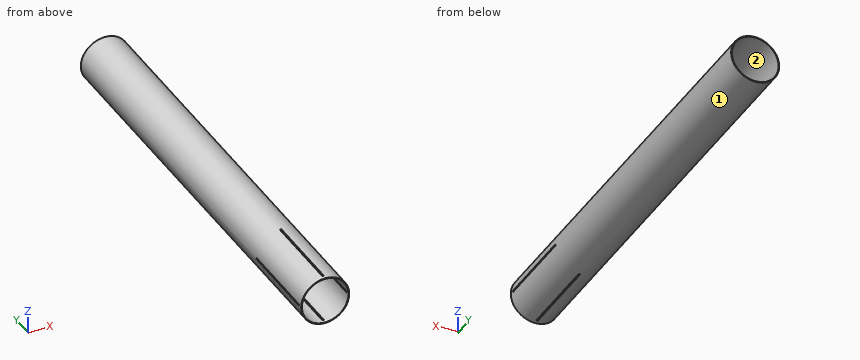
```python
from build123d import *

# Parameters (mm, degrees)
BOSS_EXTRUDE1_DEPTH      = 725
BOSS_EXTRUDE1_DEPTH_BACK = 725
SKETCH1_R                = 80.75
SKETCH1_R_2              = 78.35
SKETCH2_W                = 5.5
SKETCH2_H                = 280
CUT_EXTRUDE1_DEPTH       = 734.938774694
CIRPATTERN1_START        = -711
CIRPATTERN1_DEPTH        = 280


# Read off the part's stored shape, not the designer's step: CirPattern1
with BuildPart() as part:
    # Sketch1 → Boss-Extrude1 (new, two sides: drawn at the far end of the back side and taken through both)
    with BuildSketch(Plane(origin=(0, 0, 0), x_dir=(1, 0, 0), z_dir=(0, 1, 0)).offset(-BOSS_EXTRUDE1_DEPTH_BACK)):
        with Locations(Location((0, 0, 0), (0, 0, 270))):
            Circle(SKETCH1_R)
        with Locations(Location((0, 0, 0), (0, 0, 270))):
            Circle(SKETCH1_R_2, mode=Mode.SUBTRACT)
    extrude(amount=BOSS_EXTRUDE1_DEPTH + BOSS_EXTRUDE1_DEPTH_BACK)

    # Sketch2 → Cut-Extrude1 (cut, symmetric)
    with BuildSketch(Plane.XY):
        with Locations((0, -571)):
            Rectangle(SKETCH2_W, SKETCH2_H)
    extrude(amount=CUT_EXTRUDE1_DEPTH, both=True, mode=Mode.SUBTRACT)

    # CirPattern1 outline → CirPattern1 (cut)
    with BuildSketch(Plane(origin=(0, 0, 0), x_dir=(1, 0, 0), z_dir=(0, 1, 0)).offset(CIRPATTERN1_START)):
        with BuildLine():
            ThreePointArc((78.301724119, 2.75), (78.35, 0), (78.301724119, -2.75))
            Line((78.301724119, -2.75), (80.703159789, -2.75))
            ThreePointArc((80.703159789, -2.75), (80.75, 0), (80.703159789, 2.75))
            Line((80.703159789, 2.75), (78.301724119, 2.75))
        make_face()
        with BuildLine():
            Line((-80.703159789, -2.75), (-78.301724119, -2.75))
            ThreePointArc((-78.301724119, -2.75), (-78.35, 0), (-78.301724119, 2.75))
            Line((-78.301724119, 2.75), (-80.703159789, 2.75))
            ThreePointArc((-80.703159789, 2.75), (-80.75, 0), (-80.703159789, -2.75))
        make_face()
    extrude(amount=CIRPATTERN1_DEPTH, mode=Mode.SUBTRACT)


solid = part.part
```
Design review of the part built by this model. Coordinates are the model's own, in mm. Face numbers are marked on the shaded views. Give positions to 0.01 mm unless a question says otherwise; leave off trailing zeros. Loops run counter-clockwise (first coordinate to the right, second up) from the corner with the lowest first, then second, coordinate; pieces in that order, holes last. Notation, with made-up numbers: M 45.5,3.25 L 68.5,3.25 A15 cw 68.5,14.25 Z; hole C 59.5,46 d10. An arc over 180 degrees is marked long. Return JSON: item names as keys, results as strings. Group by question number.
Item 1: For probe 1 along Z at (x, y) = (0, -62); probe 2 along X at (y, z) = (-349, 5), list the stretches that pass through material, from the lowest coordinate up.
Item 2: We need section A-A (y = -579). Give the boundary of the cut face in (x, z), and give its area (3 significant figures).
Item 3: Insertion check: pin 1 Ø3 at (y, z) = (-425.5, 19) entering from +X; pin 2 Ø12 at (x, y) = (9.5, -331.5) entering from -Z; pin 3 Ø4 at (y, z) = (-73.5, -26) entering from +X. Each pin has a flat end and moves straight along its axis. Give the tip position at first contact, or say it passes through.
Item 4: We need section B-B (x = 53). Give the boundary of the cut face in (y, z), and give its area (3 significant figures).
Item 5: We need section D-D (y = 512). Give the boundary of the cut face in (x, z).
Item 6: Mouldability with a two-part tool opening along X and no side actions: class the marked faces 1 and 2 as released by +X, released by -X, zero draft, split by the parting line, or undercut.
Item 7: We need section C-C (z = -52). Give the boundary of the cut face in (x, y), and give its area (3 significant figures).
Output:
{
 "1": {"probe 1": "z = -80.75 to -78.35, 78.35 to 80.75", "probe 2": "x = -80.6 to -78.19, 78.19 to 80.6"},
 "2": {"outline": "M -80.7,-2.75 A80.75 ccw -2.75,-80.7 L -2.75,-78.3 A78.35 cw -78.3,-2.75 Z; M -80.7,2.75 L -78.3,2.75 A78.35 cw -2.75,78.3 L -2.75,80.7 A80.75 ccw Z; M 2.75,-80.7 A80.75 ccw 80.7,-2.75 L 78.3,-2.75 A78.35 cw 2.75,-78.3 Z; M 2.75,78.3 A78.35 cw 78.3,2.75 L 80.7,2.75 A80.75 ccw 2.75,80.7 Z", "area": "1,150 mm^2"},
 "3": {"pin 1": "stops at x = 78.83", "pin 2": "stops at z = -80.67", "pin 3": "stops at x = 77.1"},
 "4": {"outline": "M -725,-60.92 L 725,-60.92 L 725,-57.7 L -725,-57.7 Z; M -725,57.7 L 725,57.7 L 725,60.92 L -725,60.92 Z", "area": "9,330 mm^2"},
 "5": {"outline": "C 0,0 d161.5; hole C 0,0 d156.7"},
 "6": {"face 1": "split by the parting line", "face 2": "undercut"},
 "7": {"outline": "M -61.78,-725 L -58.61,-725 L -58.61,725 L -61.78,725 Z; M 58.61,-725 L 61.78,-725 L 61.78,725 L 58.61,725 Z", "area": "9,200 mm^2"}
}
